Can you work these out from the model? Positions are in its coordinate system, mm. Face numbers are marked on the shaded views. A direction names the side the tool comes from. Coordinates: 2 decimals unless noted, no trailing zeros. Order: outer loops, then holes, each group sorted by start corner. A loop starts at its lowest first (then second) coordinate and runs counter-clockwise, first axis right, second up. Notation, with made-up numbers: M -21,51 L 0,51 A30 ccw 0,87 Z; hole C 35.25,-27.5 d1. An arc over 180 degrees is marked long. Answer as a JSON object with one key per item and string values.
from build123d import *

# Parameters (mm, degrees)
BOSS_EXTRUDE1_DEPTH     = 9.5
BOSS_EXTRUDE4_DEPTH     = 19
BOSS_EXTRUDE5_DEPTH     = 2.75
CUT_EXTRUDE1_DEPTH      = 37.007750295
CUT_EXTRUDE1_DEPTH_BACK = 37.007750295
CUT_EXTRUDE2_DEPTH      = 38.700107179
CUT_EXTRUDE2_DEPTH_BACK = 38.700107179
SKETCH8_R               = 3.1


with BuildPart() as part:
    # Sketch1 → Boss-Extrude1 (new, symmetric)
    with BuildSketch(Plane(origin=(0, 0, 0), x_dir=(1, 0, 0), z_dir=(0, 1, 0))):
        with BuildLine():
            Line((-28.019427969, 0.30265419), (-26.106010807, -4.316743473))
            ThreePointArc((-26.106010807, -4.316743473), (-25.466467114, -5.100606473), (-24.5, -5.399602554))
            Line((-24.5, -5.399602554), (24.5, -5.399578272))
            ThreePointArc((24.5, -5.399578272), (25.457917057, -5.106354456), (26.098112281, -4.3358122))
            Line((26.098112281, -4.3358122), (28.019427969, 0.30265419))
            ThreePointArc((28.019427969, 0.30265419), (27.954595682, 1.785598461), (26.77403281, 2.685375236))
            ThreePointArc((26.77403281, 2.685375236), (0, 5.555679504), (-26.77374766, 2.682716614))
            ThreePointArc((-26.77374766, 2.682716614), (-27.953111468, 1.783959509), (-28.019427969, 0.30265419))
        make_face()
        with BuildLine():
            Line((-26.90965458, 0.889831635), (-24.967422855, -3.799130535))
            ThreePointArc((-24.967422855, -3.799130535), (-24.732603169, -4.057099402), (-24.386863498, -4.103492305))
            ThreePointArc((-24.386863498, -4.103492305), (0, -1.488014765), (24.386863498, -4.103492305))
            ThreePointArc((24.386863498, -4.103492305), (24.690465194, -4.081962763), (24.928721144, -3.892564732))
            Line((24.928721144, -3.892564732), (26.842138305, 0.72683293))
            ThreePointArc((26.842138305, 0.72683293), (26.889731767, 1.205196592), (26.51532004, 1.506714071))
            ThreePointArc((26.51532004, 1.506714071), (0, 4.351330223), (-26.51532004, 1.506714071))
            ThreePointArc((-26.51532004, 1.506714071), (-26.843311912, 1.281900877), (-26.90965458, 0.889831635))
        make_face(mode=Mode.SUBTRACT)
    extrude(amount=BOSS_EXTRUDE1_DEPTH, both=True)

    # Sketch5 → Boss-Extrude4 (add)
    with BuildSketch(Plane(origin=(0, 9.5, 0), x_dir=(1, 0, 0), z_dir=(0, 1, 0))):
        with BuildLine():
            Line((-28.019427969, 0.30265419), (-26.106010807, -4.316743473))
            ThreePointArc((-26.106010807, -4.316743473), (-25.466467114, -5.100606473), (-24.5, -5.399602554))
            Line((-24.5, -5.399602554), (24.5, -5.399578272))
            ThreePointArc((24.5, -5.399578272), (25.457917057, -5.106354456), (26.098112281, -4.3358122))
            Line((26.098112281, -4.3358122), (28.019427969, 0.30265419))
            ThreePointArc((28.019427969, 0.30265419), (27.954595682, 1.785598461), (26.77403281, 2.685375236))
            ThreePointArc((26.77403281, 2.685375236), (0, 5.555679504), (-26.77374766, 2.682716614))
            ThreePointArc((-26.77374766, 2.682716614), (-27.953111468, 1.783959509), (-28.019427969, 0.30265419))
        make_face()
        with BuildLine():
            Line((24.128669413, 1.955613279), (22.885024946, -3.772265844))
            ThreePointArc((22.885024946, -3.772265844), (0.000255966, -1.464252732), (-22.884068151, -3.776672574))
            Line((-22.884068151, -3.776672574), (-24.135292964, 1.986119507))
            ThreePointArc((-24.135292964, 1.986119507), (-0.001831478, 4.312848519), (24.128669413, 1.955613279))
        make_face(mode=Mode.SUBTRACT)
    extrude(amount=-BOSS_EXTRUDE4_DEPTH)

    # Sketch6 → Boss-Extrude5 (add)
    with BuildSketch(Plane(origin=(0, 9.5, 0), x_dir=(1, 0, 0), z_dir=(0, 1, 0))):
        with BuildLine():
            Line((-24.732023245, 2.377976913), (-23.267684412, -4.366358828))
            ThreePointArc((-23.267684412, -4.366358828), (0.000256463, -1.964252734), (23.268661469, -4.361858777))
            Line((23.268661469, -4.361858777), (24.725263361, 2.346842775))
            ThreePointArc((24.725263361, 2.346842775), (-0.001837352, 4.812848622), (-24.732023245, 2.377976913))
        make_face()
        with BuildLine():
            Line((-23.538121832, 1.592231661), (-22.5, -3.189067597))
            ThreePointArc((-22.5, -3.189067597), (0.000255268, -0.964252729), (22.500936706, -3.184753392))
            Line((22.500936706, -3.184753392), (23.531635738, 1.562358523))
            ThreePointArc((23.531635738, 1.562358523), (-0.001824238, 3.812848414), (-23.538121832, 1.592231661))
        make_face(mode=Mode.SUBTRACT)
    boss_extrude5 = extrude(amount=BOSS_EXTRUDE5_DEPTH)

    # Mirror1: Boss-Extrude5 across plane
    add(boss_extrude5.mirror(Plane.ZX))

    # Sketch5<2> → Cut-Extrude1 (cut, two sides: drawn at the far end of the back side and taken through both)
    with BuildSketch(Plane(origin=(0, 9.5, 0), x_dir=(1, 0, 0), z_dir=(0, 1, 0)).offset(-CUT_EXTRUDE1_DEPTH_BACK)):
        with BuildLine():
            Line((24.128669413, 1.955613279), (22.885024946, -3.772265844))
            ThreePointArc((22.885024946, -3.772265844), (0.000255966, -1.464252732), (-22.884068151, -3.776672574))
            Line((-22.884068151, -3.776672574), (-24.135292964, 1.986119507))
            ThreePointArc((-24.135292964, 1.986119507), (-0.001831478, 4.312848519), (24.128669413, 1.955613279))
        make_face()
    extrude(amount=CUT_EXTRUDE1_DEPTH + CUT_EXTRUDE1_DEPTH_BACK, mode=Mode.SUBTRACT)

    # Sketch8 → Cut-Extrude2 (cut, two sides: drawn at the far end of the back side and taken through both)
    with BuildSketch(Plane(origin=(0, 12.2, 0), x_dir=(1, 0, 0), z_dir=(0, 1, 0)).offset(-CUT_EXTRUDE2_DEPTH_BACK)):
        with Locations((0, 1.34568742)):
            Circle(SKETCH8_R)
    extrude(amount=CUT_EXTRUDE2_DEPTH + CUT_EXTRUDE2_DEPTH_BACK, mode=Mode.SUBTRACT)


solid = part.part
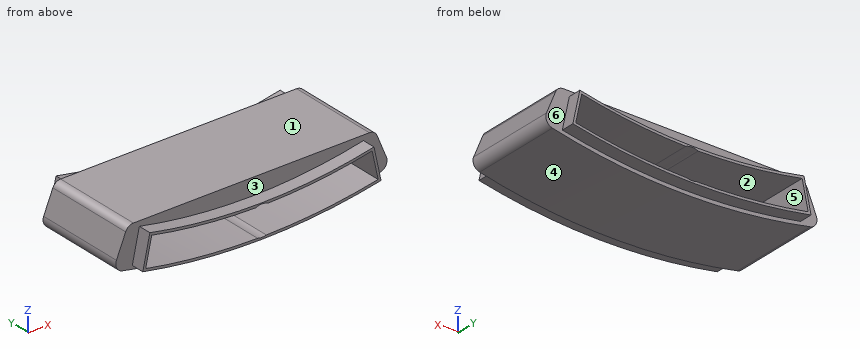
Item 1: I want a section at D-D, the plane z = -1.25. Write out the boundary of the cut face in (x, y).
Answers follow:
{"outline": "M -28.13,-9.5 L -24.49,-9.5 L -24.49,-12.25 L -23.98,-12.25 L -23.98,12.25 L -24.49,12.25 L -24.49,9.5 L -28.13,9.5 Z; M 23.98,-12.25 L 24.49,-12.25 L 24.49,-9.5 L 28.13,-9.5 L 28.13,9.5 L 24.49,9.5 L 24.49,12.25 L 23.98,12.25 Z"}
Item 2: I want a section at A-A, the plane y = -10. Write out the boundary of the cut face in (x, z).
Answers follow:
{"outline": "M -24.73,-2.38 A126 ccw 24.73,-2.35 L 23.27,4.36 A114 cw -23.27,4.37 Z; hole M -24.14,-1.99 A125.5 ccw -0.91,-4.31 A3.1 ccw 0.91,-4.31 A125.5 ccw 24.13,-1.96 L 22.89,3.77 A114.5 cw 1.29,1.47 A3.1 ccw -1.29,1.47 A114.5 cw -22.88,3.78 Z"}
Item 3: I want a section at B-B, the plane x = -20.5. Write out the boundary of the cut face in (y, z).
Answers follow:
{"outline": "M -12.25,-3.15 L -9.5,-3.15 L -9.5,-3.88 L 9.5,-3.88 L 9.5,-3.15 L 12.25,-3.15 L 12.25,-2.64 L -12.25,-2.64 Z; M -12.25,3.32 L 12.25,3.32 L 12.25,3.82 L 9.5,3.82 L 9.5,5.4 L -9.5,5.4 L -9.5,3.82 L -12.25,3.82 Z"}
Item 4: Please list where these lines run through material, in increasing order: line 1 (Z direction, x = 1.5, y = -2.75); line 2 (Y direction, x = -8.5, z = 3); line 3 (X direction, y = -7.75, z = -1).
Answers follow:
{"line 1": "z = -5.55 to -4.3, 1.47 to 5.4", "line 2": "y = -9.5 to 9.5", "line 3": "x = -28.15 to -23.92, 23.92 to 28.15"}
Item 5: I want a section at C-C, the plane z = 2.75. Write out the boundary of the cut face in (x, y), plus the area to 3 significant figures.
Answers follow:
{"outline": "M -26.75,-9.5 L -23.62,-9.5 L -23.62,-12.25 L -23.11,-12.25 L -23.11,12.25 L -23.62,12.25 L -23.62,9.5 L -26.75,9.5 Z; M -17.1,-12.25 L -13.35,-12.25 L -13.35,-9.5 L 13.37,-9.5 L 13.37,-12.25 L 17.12,-12.25 L 17.12,12.25 L 13.37,12.25 L 13.37,9.5 L -13.35,9.5 L -13.35,12.25 L -17.1,12.25 Z; M 23.11,-12.25 L 23.62,-12.25 L 23.62,-9.5 L 26.75,-9.5 L 26.75,9.5 L 23.62,9.5 L 23.62,12.25 L 23.11,12.25 Z", "area": "836 mm^2"}
Item 6: I'm going to push flat-ended pins straight in: pin 1 (1 mm diameter, centred on x = -13.5, z = 3.5, fed in from +Y); pin 2 (2 mm diameter, centred on x = -3, y = 0.5, fed in from -Z); pin 3 (3 mm diameter, centred on y = -9, z = -3.5, fed in from +X). Where does each tip first touch, or does it pass through?
Answers follow:
{"pin 1": "stops at y = 9.5", "pin 2": "stops at z = -5.54", "pin 3": "stops at x = 27.82"}
Item 7: If we mould it in two halves opening along Z, with no side actions, what happens to the marked faces 4, 5 and 6? For each: pulls with the +Z half, pulls with the -Z half, needs draft (parallel to the pull), parting line crosses it, or undercut.
Answers follow:
{"face 4": "pulls with the -Z half", "face 5": "undercut", "face 6": "needs draft"}
Item 8: Which directions (+Z, -Z, +X, -X, +Y, -Y) give clear straight access to the entire face, cutting with the end or side of a thin tool? Please do the marked faces 1, 2 and 3.
Answers follow:
{"face 1": "+Z, +X, -X, +Y, -Y", "face 2": "+Y, -Y", "face 3": "-Y"}
